Could you check a few things on this model? Use its own coordinates, in mm. A direction names the side the tool comes from. Give positions to 0.01 mm unless a question says otherwise; leave off trailing zeros. Write each loop counter-clockwise with the first axis right and the second up, starting at its lowest first coordinate (ties: lowest second). Pieces come first, ordered by that corner, then holes. Notation, with made-up numbers: (20.5, 26.5) - (37.5, 26.5) arc R8 cw to (37.5, 33.5) - close; hole circle Ø2 at (-27.5, 5). An arc over 180 degrees is marked (long way). Use one line per item in the form item = value.
```python
from build123d import *

# Parameters (mm, degrees)
PAD_DEPTH       = 17
POCKET_DEPTH    = 15
SKETCH002_R     = 3
PAD001_DEPTH    = 4
POCKET002_DEPTH = 5
POCKET003_DEPTH = 5
SKETCH006_R     = 1.99
PAD002_DEPTH    = 8
FILLET_R        = 3
FILLET001_R     = 2
FILLET002_R     = 2
SKETCH007_R     = 1
POCKET004_DEPTH = 4.5


with BuildPart() as part:
    # Sketch → Pad (new body)
    with BuildSketch(Plane.XY):
        with BuildLine():
            Line((-44.5, 38), (44.5, 38))
            ThreePointArc((49.5, 33), (48.035534, 36.535534), (44.5, 38))
            Line((49.5, 33), (49.5, -33))
            ThreePointArc((44.5, -38), (48.035534, -36.535534), (49.5, -33))
            Line((44.5, -38), (-44.5, -38))
            ThreePointArc((-49.5, -33), (-48.035534, -36.535534), (-44.5, -38))
            Line((-49.5, -33), (-49.5, 33))
            ThreePointArc((-44.5, 38), (-48.035534, 36.535534), (-49.5, 33))
        make_face()
    extrude(amount=PAD_DEPTH)

    # Sketch001 (on Face10 of Pad) → Pocket (cut)
    with BuildSketch(Plane.XY.offset(17)):
        with BuildLine():
            Line((-44.5, 36), (44.5, 36))
            ThreePointArc((47.5, 33), (46.62132, 35.12132), (44.5, 36))
            Line((47.5, 33), (47.5, -33))
            ThreePointArc((44.5, -36), (46.62132, -35.12132), (47.5, -33))
            Line((44.5, -36), (-44.5, -36))
            ThreePointArc((-47.5, -33), (-46.62132, -35.12132), (-44.5, -36))
            Line((-47.5, -33), (-47.5, 33))
            ThreePointArc((-44.5, 36), (-46.62132, 35.12132), (-47.5, 33))
        make_face()
    extrude(amount=-POCKET_DEPTH, mode=Mode.SUBTRACT)

    # Sketch002 (on Face19 of Pocket) → Pad001 (join)
    with BuildSketch(Plane.XY.offset(2)):
        with Locations((-41.25, 32.25)):
            Circle(SKETCH002_R)
        with Locations((41.25, -32.25)):
            Circle(SKETCH002_R)
    extrude(amount=PAD001_DEPTH)

    # Sketch004 → Pocket002 (cut)
    with BuildSketch(Plane.XZ.offset(38)):
        with BuildLine():
            Line((23.7, 14.6), (31.7, 14.6))
            ThreePointArc((33.2, 13.1), (32.76066, 14.16066), (31.7, 14.6))
            Line((33.2, 13.1), (33.2, 8.1))
            ThreePointArc((31.7, 6.6), (32.76066, 7.03934), (33.2, 8.1))
            Line((31.7, 6.6), (23.7, 6.6))
            ThreePointArc((22.2, 8.1), (22.63934, 7.03934), (23.7, 6.6))
            Line((22.2, 8.1), (22.2, 13.1))
            ThreePointArc((23.7, 14.6), (22.63934, 14.16066), (22.2, 13.1))
        make_face()
    extrude(amount=-POCKET002_DEPTH, mode=Mode.SUBTRACT)

    # Sketch005 (on Face1 of Pocket002) → Pocket003 (cut)
    with BuildSketch(Plane(origin=(-49.5, 0, 0), x_dir=(0, -1, 0), z_dir=(-1, 0, 0))):
        with BuildLine():
            Line((-23, 17), (-17, 17))
            Line((-17, 17), (-17, 10))
            ThreePointArc((-23, 10), (-20, 7), (-17, 10))
            Line((-23, 10), (-23, 17))
        make_face()
    extrude(amount=-POCKET003_DEPTH, mode=Mode.SUBTRACT)

    # Sketch006 (on Face30 of Pocket003) → Pad002 (join)
    with BuildSketch(Plane.XY.offset(9)):
        with BuildLine():
            Line((44.5, 36), (35.5, 36))
            Line((35.5, 36), (35.5, 27))
            ThreePointArc((35.5, 27), (36.37868, 24.87868), (38.5, 24))
            Line((38.5, 24), (47.5, 24))
            Line((47.5, 24), (47.5, 33))
            ThreePointArc((47.5, 33), (46.62132, 35.12132), (44.5, 36))
        make_face()
        with Locations((41.5, 30)):
            Circle(SKETCH006_R, mode=Mode.SUBTRACT)
        with BuildLine():
            Line((-38.5, -24), (-47.5, -24))
            Line((-47.5, -24), (-47.5, -33))
            ThreePointArc((-47.5, -33), (-46.62132, -35.12132), (-44.5, -36))
            Line((-44.5, -36), (-35.5, -36))
            Line((-35.5, -36), (-35.5, -27))
            ThreePointArc((-35.5, -27), (-36.37868, -24.87868), (-38.5, -24))
        make_face()
        with Locations((-41.5, -30)):
            Circle(SKETCH006_R, mode=Mode.SUBTRACT)
    extrude(amount=PAD002_DEPTH)

    # Fillet
    fillet_edges = [part.edges().sort_by_distance(p)[0] for p in [
        (47.5, 24, 13),
        (35.5, 36, 13),
        (-35.5, -36, 13),
        (-47.5, -24, 13),
    ]]
    fillet(fillet_edges, radius=FILLET_R)

    # Fillet001
    fillet001_edges = [part.edges().sort_by_distance(p)[0] for p in [
        (40, 36, 9),
        (47.5, 28.5, 9),
        (47.5, 22.5, 9),
        (34, 36, 9),
    ]]
    fillet(fillet001_edges, radius=FILLET001_R)

    # Fillet002
    fillet002_edges = [part.edges().sort_by_distance(p)[0] for p in [
        (-46.62132, -35.12132, 9),
        (-47.5, -28.5, 9),
        (-47.5, -22.5, 9),
        (-40, -36, 9),
        (-34, -36, 9),
    ]]
    fillet(fillet002_edges, radius=FILLET002_R)

    # Sketch007 (on Face54 of Fillet002) → Pocket004 (cut)
    with BuildSketch(Plane.XY.offset(6)):
        with Locations((41.25, -32.25)):
            Circle(SKETCH007_R)
        with Locations((-41.25, 32.25)):
            Circle(SKETCH007_R)
    extrude(amount=-POCKET004_DEPTH, mode=Mode.SUBTRACT)


solid = part.part
```
1. Which directions (+Z, -Z, +X, -X, +Y, -Y) give clear straight access to the entire face, cutting with the end or side of a thin tool? Please do faces 4 (the face through (41, -34, 6)), 5 (the face through (22.2, -37, 11)), 6 (the face through (-49, 20, 7)), 7 (the face through (46.93, 28.25, 8.4)).
Response values:
face_4 = +Z
face_5 = -Y
face_6 = +Z, -X
face_7 = none
2. If we mould it in two halves opening along Y, with no side actions, what happens to faces 1 (the face through (-1, 38, 8)), 2 (the face through (33.2, -37, 11)), 3 (the face through (46.6, 23.14, 13.18))? For each: pulls with the +Y half, pulls with the -Y half, needs draft (parallel to the pull), parting line crosses it, or undercut.
Response values:
face_1 = pulls with the +Y half
face_2 = needs draft
face_3 = undercut
3. Imagine slicing it at A-A, the plane y = -2.5. List the corners of the cut face in (x, z) for me, and give its area (3 significant figures).
Response values:
outline = (-49.5, 0) - (49.5, 0) - (49.5, 17) - (47.5, 17) - (47.5, 2) - (-47.5, 2) - (-47.5, 17) - (-49.5, 17) - close
area = 258 mm²
4. If I drill on line 1 (Y direction, x = -41.25, z = 2.8); line 2 (Y direction, x = 41.5, z = 12); line 3 (Y direction, x = 41.25, z = 3.55), over which ranges is the centre line in solid material (lowest first)? Write a range as from..to.
Response values:
line_1 = -38..-36, 29.25..31.25, 33.25..35.25, 36..38
line_2 = -38..-36, 24..28.01, 31.99..38
line_3 = -38..-36, -35.25..-33.25, -31.25..-29.25, 36..38
5. For pin 1 (1.6 mm diameter, centred on x = 28.5, y = -36.5, fed in from -Z); pin 2 (10 mm diameter, centred on x = -14.5, y = 3, fed in from +Z); pin 3 (2 mm diameter, centred on y = -37, z = 10.5, fed in from +X); pin 4 (3 mm diameter, centred on x = -41.25, y = 32.25, fed in from +Z), each with a flat end and sliding along its axis, tell me the tip position at first contact or that it passes through.
Response values:
pin_1 = 0
pin_2 = 2
pin_3 = 48.5
pin_4 = 6
6. Imagine slicing it at B-B, the plane x = -15. List the corners of the cut face in (y, z) for me.
Response values:
outline = (-38, 0) - (38, 0) - (38, 17) - (36, 17) - (36, 2) - (-36, 2) - (-36, 17) - (-38, 17) - close
